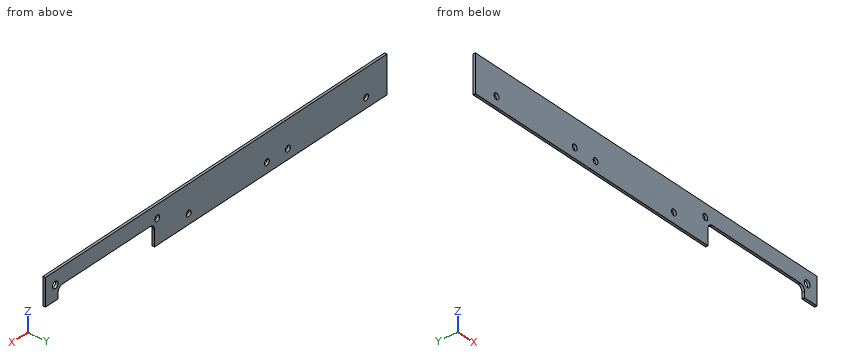
```python
from build123d import *

# Parameters (mm, degrees)
SKETCH_1_R      = 1.75
SKETCH_1_R_2    = 2
EXTRUDE_1_DEPTH = 1.5


with BuildPart() as part:
    # Эскиз1 → Бобышка-Вытянуть1 (new body)
    with BuildSketch(Plane(origin=(0, 0, 0), x_dir=(1, 0, 0), z_dir=(0, 1, 0))):
        with BuildLine():
            Line((166.5, 12.5), (166.5, 22))
            Line((166.5, 22), (0, 22))
            Line((0, 22), (0, 0))
            Line((0, 0), (244.5, 0))
            Line((244.5, 0), (244.5, 16))
            Line((244.5, 16), (235.5, 16))
            Line((235.5, 16), (235.5, 12.5))
            ThreePointArc((235.5, 12.5), (234.621320344, 10.378679656), (232.5, 9.5))
            Line((232.5, 9.5), (169.5, 9.5))
            ThreePointArc((169.5, 9.5), (167.378679656, 10.378679656), (166.5, 12.5))
        make_face()
        with Locations((164.5, 7.5)):
            Circle(SKETCH_1_R, mode=Mode.SUBTRACT)
        with Locations((237.5, 7.5)):
            Circle(SKETCH_1_R_2, mode=Mode.SUBTRACT)
        with Locations((15, 16)):
            Circle(SKETCH_1_R, mode=Mode.SUBTRACT)
        with Locations((71, 16)):
            Circle(SKETCH_1_R, mode=Mode.SUBTRACT)
        with Locations((86, 16)):
            Circle(SKETCH_1_R, mode=Mode.SUBTRACT)
        with Locations((142, 16)):
            Circle(SKETCH_1_R, mode=Mode.SUBTRACT)
    extrude(amount=EXTRUDE_1_DEPTH)


solid = part.part
```
Part model, mm, in its own coordinate system. Round coordinates to 2 decimals unless told otherwise and drop trailing zeros. Write each loop counter-clockwise with the first axis right and the second up, starting at its lowest first coordinate (ties: lowest second). Pieces come first, ordered by that corner, then holes.
Item 1: Probe L1, parallel to X at y = 0.8, z = -7.5; L2, parallel to Z at x = 86, y = 1; L3, parallel to Z at x = 164.5, y = 0.6. List the from-to ranges inside material, lowest first.
Results:
L1: x = 0 to 162.75, 166.25 to 235.5, 239.5 to 244.5
L2: z = -22 to -17.75, -14.25 to 0
L3: z = -22 to -9.25, -5.75 to 0
Item 2: Cut at B-B, the plane y = 0.6. Give the cut face in (x, z), plus the area to 3 significant figures.
Results:
outline: (0, -22) - (166.5, -22) - (166.5, -12.5) arc R3 cw to (169.5, -9.5) - (232.5, -9.5) arc R3 cw to (235.5, -12.5) - (235.5, -16) - (244.5, -16) - (244.5, 0) - (0, 0) - close; hole circle Ø3.5 at (15, -16); hole circle Ø3.5 at (71, -16); hole circle Ø3.5 at (86, -16); hole circle Ø3.5 at (142, -16); hole circle Ø3.5 at (164.5, -7.5); hole circle Ø4 at (237.5, -7.5)
area: 4,410 mm2
Item 3: Cut at C-C, the plane x = 173. Give the cut face in (y, z), plus the area to 4 significant figures.
Results:
outline: (0, -9.5) - (1.5, -9.5) - (1.5, 0) - (0, 0) - close
area: 14.25 mm2
Item 4: Cut at A-A, the plane x = 237.5. Give the cut face in (y, z), plus the area to 3 significant figures.
Results:
outline: (0, -16) - (1.5, -16) - (1.5, -9.5) - (0, -9.5) - close; (0, -5.5) - (1.5, -5.5) - (1.5, 0) - (0, 0) - close
area: 18.0 mm2
Item 5: Drop flat-ended pins along their axis: pin 1 Ø2 at (x, z) = (15, -16) entering from -Y; pin 2 Ø0.8 at (x, y) = (240, 0.5) entering from -Z. Give the stop position or say it passes through.
Results:
pin 1: passes through
pin 2: stops at z = -16
